Geometry: final body of the model. Coordinates: model frame, mm. A direction names the side the tool comes from. Coordinates: 2 decimals unless noted, no trailing zeros. Write each loop counter-clockwise with the first axis right and the second up, starting at its lowest first coordinate (ties: lowest second). Pieces come first, ordered by that corner, then holes.
from build123d import *

# Parameters (mm, degrees)
SKETCH1_R           = 6.35
SKETCH1_R_2         = 3.175
BOSS_EXTRUDE4_DEPTH = 9.652
BOSS_EXTRUDE5_START = -1.778
SKETCH2_W           = 19.05
SKETCH2_H           = 6.35
BOSS_EXTRUDE5_DEPTH = 105.33369205
BOSS_EXTRUDE6_START = 21.082
BOSS_EXTRUDE6_DEPTH = 12.7
BOSS_EXTRUDE7_START = -1.778
BOSS_EXTRUDE7_DEPTH = 12.7


with BuildPart() as part:
    # Sketch1 → Boss-Extrude4 (new body)
    # profile 1 of 5: a face of its own
    with BuildSketch(Plane(origin=(0, 0, 0), x_dir=(1, 0, 0), z_dir=(0, 1, 0))):
        Polygon((-1.790492958, -55.894278169), (-1.790492958, 1.255721831), (96.761507042, 1.255721831), (103.496699133, -5.47947026), (103.496699133, -49.159086078), (96.761507042, -55.894278169), align=None)
        with Locations((68.313507042, -43.194278169)):
            Circle(SKETCH1_R, mode=Mode.SUBTRACT)
        with Locations((33.261507042, -43.194278169)):
            Circle(SKETCH1_R, mode=Mode.SUBTRACT)
        with Locations((68.313507042, -11.444278169)):
            Circle(SKETCH1_R, mode=Mode.SUBTRACT)
        with Locations((33.261507042, -11.444278169)):
            Circle(SKETCH1_R, mode=Mode.SUBTRACT)
    # profile 2 of 5: a face of its own
    with BuildSketch(Plane(origin=(0, 0, 0), x_dir=(1, 0, 0), z_dir=(0, 1, 0))):
        with Locations((68.313507042, -43.194278169)):
            Circle(SKETCH1_R)
        with Locations(Location((68.313507042, -43.194278169, 0), (0, 0, 270))):
            Circle(SKETCH1_R_2, mode=Mode.SUBTRACT)
    # profile 3 of 5: a face of its own
    with BuildSketch(Plane(origin=(0, 0, 0), x_dir=(1, 0, 0), z_dir=(0, 1, 0))):
        with Locations((33.261507042, -43.194278169)):
            Circle(SKETCH1_R)
        with Locations(Location((33.261507042, -43.194278169, 0), (0, 0, 270))):
            Circle(SKETCH1_R_2, mode=Mode.SUBTRACT)
    # profile 4 of 5: a face of its own
    with BuildSketch(Plane(origin=(0, 0, 0), x_dir=(1, 0, 0), z_dir=(0, 1, 0))):
        with Locations((33.261507042, -11.444278169)):
            Circle(SKETCH1_R)
        with Locations(Location((33.261507042, -11.444278169, 0), (0, 0, 270))):
            Circle(SKETCH1_R_2, mode=Mode.SUBTRACT)
    # profile 5 of 5: a face of its own
    with BuildSketch(Plane(origin=(0, 0, 0), x_dir=(1, 0, 0), z_dir=(0, 1, 0))):
        with Locations((68.313507042, -11.444278169)):
            Circle(SKETCH1_R)
        with Locations(Location((68.313507042, -11.444278169, 0), (0, 0, 270))):
            Circle(SKETCH1_R_2, mode=Mode.SUBTRACT)
    extrude(amount=-BOSS_EXTRUDE4_DEPTH)

    # Cut-Extrude4 cone 1 section (on through the dimple's axis) → Cut-Extrude4 (revolve, cut)
    with BuildSketch(Plane(origin=(33.261507042, 0, 11.444278169), x_dir=(0, 0, 1), z_dir=(1, 0, 0))):
        Polygon((0, 0), (6.35, 0), (0, 6.35), align=None)
    revolve(axis=Axis((33.261507042, 0, 11.444278169), (0, -1, 0)), mode=Mode.SUBTRACT)

    # Cut-Extrude4 cone 2 section (on through the dimple's axis) → Cut-Extrude4 cone 2 (revolve, cut)
    with BuildSketch(Plane(origin=(68.313507042, 0, 11.444278169), x_dir=(0, 0, 1), z_dir=(1, 0, 0))):
        Polygon((0, 0), (6.35, 0), (0, 6.35), align=None)
    revolve(axis=Axis((68.313507042, 0, 11.444278169), (0, -1, 0)), mode=Mode.SUBTRACT)

    # Cut-Extrude4 cone 3 section (on through the dimple's axis) → Cut-Extrude4 cone 3 (revolve, cut)
    with BuildSketch(Plane(origin=(33.261507042, 0, 43.194278169), x_dir=(0, 0, 1), z_dir=(1, 0, 0))):
        Polygon((0, 0), (6.35, 0), (0, 6.35), align=None)
    revolve(axis=Axis((33.261507042, 0, 43.194278169), (0, -1, 0)), mode=Mode.SUBTRACT)

    # Cut-Extrude4 cone 4 section (on through the dimple's axis) → Cut-Extrude4 cone 4 (revolve, cut)
    with BuildSketch(Plane(origin=(68.313507042, 0, 43.194278169), x_dir=(0, 0, 1), z_dir=(1, 0, 0))):
        Polygon((0, 0), (6.35, 0), (0, 6.35), align=None)
    revolve(axis=Axis((68.313507042, 0, 43.194278169), (0, -1, 0)), mode=Mode.SUBTRACT)

    # Sketch2 → Boss-Extrude5 (add)
    with BuildSketch(Plane(origin=(0, 0, 0), x_dir=(0, 0, -1), z_dir=(1, 0, 0)).offset(BOSS_EXTRUDE5_START)):
        with Locations((-27.319278169, -12.827)):
            Rectangle(SKETCH2_W, SKETCH2_H)
    extrude(amount=BOSS_EXTRUDE5_DEPTH)

    # Sketch4 → Boss-Extrude6 (add)
    with BuildSketch(Plane.XY.offset(BOSS_EXTRUDE6_START)):
        Polygon((10.909507042, 0), (10.909507042, 41.148), (75.048699133, 0), align=None)
    extrude(amount=BOSS_EXTRUDE6_DEPTH)

    # Sketch5 → Boss-Extrude7 (add)
    with BuildSketch(Plane(origin=(0, 0, 0), x_dir=(0, 0, -1), z_dir=(1, 0, 0)).offset(BOSS_EXTRUDE7_START)):
        Polygon((-14.81428613, 41.148), (-40.21428613, 41.148), (-55.894278169, 0), (1.255721831, 0), align=None)
    extrude(amount=BOSS_EXTRUDE7_DEPTH)


solid = part.part
Item 1: Section D-D, the plane y = 16. Output: boundary loops of the cut face in (x, z).
Derived:
outline: (-1.78, 4.99) - (10.92, 4.99) - (10.92, 21.08) - (50.11, 21.08) - (50.11, 33.78) - (10.92, 33.78) - (10.92, 49.8) - (-1.78, 49.8) - close
Item 2: Pull-direction query (X, two-part tool) for faces 1 (the flat face through (47, -5, -1.256)), 2 (the flat face through (-1.778, 16, 28)), 3 (the conical face through (71.27, -3.02, 12.98)); classes: released by +X, released by -X, zero draft, split by the parting line, or undercut.
Derived:
face 1: zero draft
face 2: released by -X
face 3: undercut
Item 3: Set-up query: faces 4 (the flat face through (29, 12, 21.082)), 5 (the flat face through (100.176, -4.758, 52.48)), 6 (the flat face through (56.6, 0, 20.6)). Return all of +Z, -Z, +X, -X, +Y, -Y with unobstructed straight access to the full face (end or side cutting, diameter ignored); none if empty.
Derived:
face 4: -Z, +X, +Y
face 5: +Z, +X, +Y, -Y
face 6: +X, +Y
Item 4: Section B-B, the plane x = 9. Output: boundary loops of the cut face in (y, z), plus the area to 3 significant figures.
Derived:
outline: (-16, 17.79) - (-9.65, 17.79) - (-9.65, -1.26) - (0, -1.26) - (41.15, 14.81) - (41.15, 40.21) - (0, 55.89) - (-9.65, 55.89) - (-9.65, 36.84) - (-16, 36.84) - close
area: 2,370 mm2
Item 5: Material intervals for probe 1 along Z at (x, y) = (36, -9.5); probe 2 along Z at (x, y) = (69.5, -5); probe 3 along Y at (x, z) = (18.5, 19.5), sorted ascending.
Derived:
probe 1: z = -1.26 to 9.84, 13.05 to 41.59, 44.8 to 55.89
probe 2: z = -1.26 to 8.5, 14.39 to 40.25, 46.14 to 55.89
probe 3: y = -16 to 0
Item 6: Section A-A, the plane y = -5.5. State how many separate pieces and enclosed holes the cut face has, plus the area to 3 significant figures.
Derived:
separate pieces: 1
enclosed holes: 4
area: 5,850 mm2
Item 7: Pin query (flat end, axial travel): pin 1 (1.5 mm diameter, centred on y = -7, z = 49.5, fed in from +X); pin 2 (8 mm diameter, centred on y = 30, z = 37, fed in from -X); pin 3 (5 mm diameter, centred on x = 67.5, y = -12.5, fed in from -Z). Return the tip coordinate at first contact, or that it passes through.
Derived:
pin 1: stops at x = 103.5
pin 2: stops at x = -1.78
pin 3: stops at z = 17.79
